Build history of the part. All positions in model axes, mm. A direction names the side the tool comes from. Coordinates: 2 decimals unless noted, no trailing zeros. Order: outer loops, then holes, each group sorted by start corner. A loop starts at its lowest first (then second) coordinate and runs counter-clockwise, first axis right, second up. Notation, with made-up numbers: M 86.5,84.5 L 92.5,84.5 A22 ccw 92.5,119.5 Z; hole C 43,57.5 d7. An arc over 180 degrees is marked long. Write item = value, one per line. Start each with the question number.
Q1. Drill centre lines: probe 1 along X at (y, z) = (16.5, -59.5); probe 2 along Z at (x, y) = (27, 20); probe 3 along Z at (x, y) = (25, 19.5). Where is each one in solid material? Low to high.
Q2. Band-saw the part on B-B on x = 18.5. Write the cut outline in (y, z).
Q3. Pull direction Z, two halves, no side cores. Call faces 1 (the face through (18.97, 14.4, -66.49)), 2 (the face through (46.6, 15.5, -27.7)), 3 (the face through (54.084, 14.297, -27.667)), 4 (the face through (46.744, 14.486, -28.154)): released by +Z, released by -Z, zero draft, split by the parting line, or undercut.
Q4. Pin check, flat tips, straight feed: P1, Ø3, axis at y = 5, z = -20.5, coming from the -X side; P2, Ø4, axis at x = 46.5, z = -28.5, coming from the +Y side; P3, Ø12, axis at x = 34, y = 13.5, coming from the -Z side. Stop position of each tip, or through.
Q5. Band-saw the part on D-D on y = 2.25. Write the cut outline in (x, z).
Q6. 3-axis set-ups, long thin cutter, end or side, ignore diameter. For faces 5 (the face through (36.227, 3.802, -61.301)), 6 (the face through (46.6, 13.5, -27.7)), 7 (the face through (36.29, 25.3, -61.13)), 8 (the face through (44.295, 14.297, -54.227)): which of +Z, -Z, +X, -X, +Y, -Y reach the whole face in a straight line?
Q7. Band-saw the part on A-A on z = -58.5. Write the cut outline in (x, y), plus the area to 3 significant figures.
Q8. Band-saw the part on C-C on y = 19. Write the cut outline in (x, z).
```python
from build123d import *

# Parameters (mm, degrees)
SKETCH2_R                = 5.5
BOSS_EXTRUDE1_DEPTH      = 29
SKETCH3_R                = 12
CUT_EXTRUDE5_DEPTH       = 7
CUT_EXTRUDE5_DEPTH_BACK  = 0.5
SKETCH6_R                = 12
CUT_EXTRUDE6_DEPTH       = 7
CUT_EXTRUDE6_DEPTH_BACK  = 0.5
SKETCH9_R                = 4
SKETCH9_R_2              = 2
BOSS_EXTRUDE2_DEPTH      = 1
BOSS_EXTRUDE2_DEPTH_BACK = 1


with BuildPart() as part:
    # Sketch2 → Boss-Extrude1 (new body)
    with BuildSketch(Plane(origin=(0, 0, 0), x_dir=(1, 0, 0), z_dir=(0, 1, 0))):
        with BuildLine():
            ThreePointArc((50.009794046, 41.311227393), (41.887297641, 57.884223181), (28.818508763, 70.916716976))
            ThreePointArc((28.818508763, 70.916716976), (13.814285335, 58.864855467), (32.908133208, 61.2729792))
            ThreePointArc((32.908133208, 61.2729792), (40.45496434, 51.34849017), (45.618872448, 40.00017771))
            Line((45.618872448, 40.00017771), (51.710808427, 16.848599978))
            Line((51.710808427, 16.848599978), (58.045348615, 14.398829975))
            Line((58.045348615, 14.398829975), (50.009794046, 41.311227393))
        make_face()
        with Locations((23.020672213, 62.769012309)):
            Circle(SKETCH2_R, mode=Mode.SUBTRACT)
    extrude(amount=BOSS_EXTRUDE1_DEPTH)

    # Sketch3 → Cut-Extrude5 (cut, two sides)
    with BuildSketch(Plane(origin=(0, 7, 0), x_dir=(-1, 0, 0), z_dir=(0, -1, 0))) as cut_extrude5_sk:
        Polygon((-39.457331724, 64.63900974), (-16.53662743, 40.953334568), (-1.019451578, 59.252301049), (-23.940155872, 82.937976221), align=None)
        with Locations((-23.020672213, 62.769012309)):
            Circle(SKETCH3_R, mode=Mode.SUBTRACT)
        with BuildLine():
            ThreePointArc((-11.020672213, 62.769012309), (-24.609375035, 74.663381706), (-34.600009437, 59.619575938))
            Line((-34.600009437, 59.619575938), (-26.548423191, 51.29927068))
            ThreePointArc((-26.548423191, 51.29927068), (-15.890911057, 53.116732482), (-11.020672213, 62.769012309))
        make_face()
        with BuildLine():
            Line((-26.548423191, 51.29927068), (-34.600009437, 59.619575938))
            ThreePointArc((-34.600009437, 59.619575938), (-31.644064723, 54.424127551), (-26.548423191, 51.29927068))
        make_face()
    extrude(amount=CUT_EXTRUDE5_DEPTH, mode=Mode.SUBTRACT)
    extrude(cut_extrude5_sk.sketch, amount=-CUT_EXTRUDE5_DEPTH_BACK, mode=Mode.SUBTRACT)

    # Sketch6 → Cut-Extrude6 (cut, two sides)
    with BuildSketch(Plane(origin=(0, 22, 0), x_dir=(1, 0, 0), z_dir=(0, 1, 0))) as cut_extrude6_sk:
        Polygon((38.61882347, 63.432982973), (15.193844621, 40.271001155), (3.602276136, 63.900303012), (27.027254985, 87.06228483), align=None)
        with Locations((23.020672213, 62.769012309)):
            Circle(SKETCH6_R, mode=Mode.SUBTRACT)
        with BuildLine():
            ThreePointArc((26.262238297, 51.21512771), (31.457917246, 54.235965008), (34.537222393, 59.397206866))
            Line((34.537222393, 59.397206866), (26.262238297, 51.21512771))
        make_face()
        with BuildLine():
            Line((26.262238297, 51.21512771), (34.537222393, 59.397206866))
            ThreePointArc((34.537222393, 59.397206866), (34.899194894, 61.065868475), (35.020672213, 62.769012309))
            ThreePointArc((35.020672213, 62.769012309), (13.457754431, 70.018191814), (26.262238297, 51.21512771))
        make_face()
    extrude(amount=CUT_EXTRUDE6_DEPTH, mode=Mode.SUBTRACT)
    extrude(cut_extrude6_sk.sketch, amount=-CUT_EXTRUDE6_DEPTH_BACK, mode=Mode.SUBTRACT)

    # Sketch9 → Boss-Extrude2 (add, two sides)
    with BuildSketch(Plane(origin=(0, 14.5, 0), x_dir=(1, 0, 0), z_dir=(0, 1, 0))) as boss_extrude2_sk:
        with Locations((48.688174425, 28.621117181)):
            Circle(SKETCH9_R)
        with Locations((48.688174425, 28.621117181)):
            Circle(SKETCH9_R_2, mode=Mode.SUBTRACT)
    extrude(amount=BOSS_EXTRUDE2_DEPTH)
    extrude(boss_extrude2_sk.sketch, amount=-BOSS_EXTRUDE2_DEPTH_BACK)


solid = part.part
```
Recorded:
q1.probe_1 = 13.57 to 18.6, 27.44 to 32.47, 34.53 to 40.69
q1.probe_2 = -71.94 to -66.57, -58.97 to -53.59
q1.probe_3 = -72.57 to -67.9, -57.64 to -52.97
q2.outline = M 7.5,-71.69 L 21.5,-71.69 L 21.5,-65.9 L 7.5,-65.9 Z; M 7.5,-59.64 L 21.5,-59.64 L 21.5,-53.85 L 7.5,-53.85 Z
q3.face_1 = undercut
q3.face_2 = zero draft
q3.face_3 = released by -Z
q3.face_4 = undercut
q4.P1 = 50.36
q4.P2 = 15.5
q4.P3 = -71.44
q5.outline = M 34.56,-59.47 A12 cw 34.6,-59.62 L 37.81,-62.94 A56 ccw 50.01,-41.31 L 58.05,-14.4 L 51.71,-16.85 L 45.62,-40 A56 cw Z
q6.face_5 = -Z, -X, -Y
q6.face_6 = +Z, -X, -Y
q6.face_7 = -Z, -X, +Y
q6.face_8 = -Z, +X, +Y, -Y
q7.outline = M 13.98,7.5 L 19.55,7.5 L 19.55,21.5 L 13.98,21.5 Z; M 26.49,7.5 L 32.06,7.5 L 32.06,21.5 L 26.49,21.5 Z; M 35.38,0 L 41.44,0 L 41.44,29 L 35.38,29 Z
q7.area = 332 mm2
q8.outline = M 28.82,-70.92 A56 ccw 50.01,-41.31 L 58.05,-14.4 L 51.71,-16.85 L 45.62,-40 A56 cw 32.91,-61.27 A10 ccw long Z; hole C 23.02,-62.77 d11
